from build123d import *
from build123d.topology import SkipClean

# Parameters (mm, degrees)
BOSS_EXTRUDE1_DEPTH = 5
BOSS_EXTRUDE2_DEPTH = 5
SKETCH4_R           = 1.5
SKETCH4_W           = 21.014084041
SKETCH4_H           = 55
SKETCH4_W_2         = 12
SKETCH4_H_2         = 5
CUT_EXTRUDE1_DEPTH  = 5
CIRPATTERN1_COUNT   = 3
SKETCH5_R           = 188.544827525
CUT_EXTRUDE2_DEPTH  = 5
BOSS_EXTRUDE3_START = -5
BOSS_EXTRUDE3_DEPTH = 5
BOSS_EXTRUDE4_START = -5
BOSS_EXTRUDE4_DEPTH = 5
BOSS_EXTRUDE5_START = -5
BOSS_EXTRUDE5_DEPTH = 5
CUT_EXTRUDE3_DEPTH  = 5
SKETCH8_R           = 1.5
SKETCH8_W           = 5
SKETCH8_H           = 15
CUT_EXTRUDE4_DEPTH  = 10
CIRPATTERN2_COUNT   = 3


with BuildPart() as part:
    # Sketch1 → Boss-Extrude1 (new body)
    with BuildSketch(Plane.XY):
        with BuildLine():
            Line((-8.818414939, -40.273942716), (-43.818414939, -100.895720981))
            ThreePointArc((-43.818414939, -100.895720981), (55, -95.262794416), (109.287464972, -12.5))
            Line((109.287464972, -12.5), (39.287464972, -12.5))
            Line((39.287464972, -12.5), (39.287464972, 12.5))
            Line((39.287464972, 12.5), (109.287464972, 12.5))
            ThreePointArc((109.287464972, 12.5), (55, 95.262794416), (-43.818414939, 100.895720981))
            Line((-43.818414939, 100.895720981), (-8.818414939, 40.273942716))
            Line((-8.818414939, 40.273942716), (-30.469050033, 27.773942716))
            Line((-30.469050033, 27.773942716), (-65.469050033, 88.395720981))
            ThreePointArc((-65.469050033, 88.395720981), (-110, 0), (-65.469050033, -88.395720981))
            Line((-65.469050033, -88.395720981), (-30.469050033, -27.773942716))
            Line((-30.469050033, -27.773942716), (-8.818414939, -40.273942716))
        make_face()
    extrude(amount=BOSS_EXTRUDE1_DEPTH)

    # Sketch3 → Boss-Extrude2 (add)
    with BuildSketch(Plane.XY.offset(5)):
        with BuildLine():
            Line((145.507042021, -22.5), (145.507042021, 22.5))
            ThreePointArc((145.507042021, 22.5), (141.113643739, 33.106601718), (130.507042021, 37.5))
            Line((130.507042021, 37.5), (96.507042021, 37.5))
            Line((96.507042021, 37.5), (96.507042021, -37.5))
            Line((96.507042021, -37.5), (130.507042021, -37.5))
            ThreePointArc((130.507042021, -37.5), (141.113643739, -33.106601718), (145.507042021, -22.5))
        make_face()
        with BuildLine():
            Line((120.507042021, -27.5), (106.507042021, -27.5))
            Line((106.507042021, -27.5), (106.507042021, 27.5))
            Line((106.507042021, 27.5), (120.507042021, 27.5))
            ThreePointArc((120.507042021, 27.5), (131.113643739, 23.106601718), (135.507042021, 12.5))
            Line((135.507042021, 12.5), (135.507042021, -12.5))
            ThreePointArc((135.507042021, -12.5), (131.113643739, -23.106601718), (120.507042021, -27.5))
        make_face(mode=Mode.SUBTRACT)
    boss_extrude2 = extrude(amount=-BOSS_EXTRUDE2_DEPTH)

    # Sketch4 → Cut-Extrude1 (cut)
    with BuildSketch(Plane.XY.offset(5)):
        with Locations((72.5, -20.5)):
            Circle(SKETCH4_R)
        with Locations((72.5, 20.5)):
            Circle(SKETCH4_R)
        with Locations((47.5, 20.5)):
            Circle(SKETCH4_R)
        with Locations((47.5, -20.861898396)):
            Circle(SKETCH4_R)
        with Locations((106.50704202, 0)):
            Rectangle(SKETCH4_W, SKETCH4_H)
        with Locations((85, -20.5)):
            Rectangle(SKETCH4_W_2, SKETCH4_H_2)
        with Locations((60, -20.5)):
            Rectangle(SKETCH4_W_2, SKETCH4_H_2)
        with Locations((85, 20.5)):
            Rectangle(SKETCH4_W_2, SKETCH4_H_2)
        with Locations((60, 20.5)):
            Rectangle(SKETCH4_W_2, SKETCH4_H_2)
    cut_extrude1 = extrude(amount=-CUT_EXTRUDE1_DEPTH, mode=Mode.SUBTRACT)

    # CirPattern1: Boss-Extrude2, Cut-Extrude1 ×3 about axis
    cirpattern1_axis = Axis((0, 0, 0), (0, 0, 1))
    add([boss_extrude2.rotate(cirpattern1_axis, i * 360 / CIRPATTERN1_COUNT) for i in range(1, CIRPATTERN1_COUNT)])
    add([cut_extrude1.rotate(cirpattern1_axis, i * 360 / CIRPATTERN1_COUNT) for i in range(1, CIRPATTERN1_COUNT)], mode=Mode.SUBTRACT)

    # Sketch5 → Cut-Extrude2 (cut)
    with BuildSketch(Plane.XY.offset(5)):
        with Locations((130.507042021, 226.044827525)):
            Circle(SKETCH5_R)
    extrude(amount=-CUT_EXTRUDE2_DEPTH, mode=Mode.SUBTRACT)

    # Sketch5_2 → Boss-Extrude3 (add)
    with SkipClean():  # the faces are left unmerged after this step: merging them gives an invalid solid
        with BuildSketch(Plane.XY.offset(5).offset(BOSS_EXTRUDE3_START)):
            with BuildLine():
                ThreePointArc((-17.04807225, 108.670894137), (-25.34145383, 119.929803482), (-32.777568368, 131.772413763))
                Line((-32.777568368, 131.772413763), (-19.229342058, 108.30619744))
                ThreePointArc((-19.229342058, 108.30619744), (-18.139623705, 108.494027724), (-17.04807225, 108.670894137))
            make_face()
            with BuildLine():
                Line((103.4105894, 37.5), (130.507042021, 37.5))
                ThreePointArc((130.507042021, 37.5), (116.532983402, 38.018558956), (102.6357911, 39.571383414))
                ThreePointArc((102.6357911, 39.571383414), (103.02839602, 38.537638919), (103.4105894, 37.5))
            make_face()
        extrude(amount=BOSS_EXTRUDE3_DEPTH)

    # Sketch6 → Boss-Extrude4 (add)
    with SkipClean():  # the faces are left unmerged after this step: merging them gives an invalid solid
        with BuildSketch(Plane.XY.offset(5).offset(BOSS_EXTRUDE4_START)):
            with BuildLine():
                add(Edge.make_bspline(
                    [(139.712182128, -34.343369267), (99.956513164, -69.307138706), (55.000005485, -95.262791249)],
                    knots=[0.008670154, 0.008670154, 0.008670154, 0.49999997, 0.49999997, 0.49999997], degree=2))
                ThreePointArc((139.712182128, -34.343369267), (135.372710576, -36.688913613), (130.507042021, -37.5))
                Line((130.507042021, -37.5), (103.4105894, -37.5))
                ThreePointArc((103.4105894, -37.5), (84.306667329, -70.656817391), (55.000005485, -95.262791249))
            make_face()
            with BuildLine():
                ThreePointArc((-32.777568368, -131.772413763), (-35.912824062, -135.580663145), (-40.113860827, -138.165983575))
                add(Edge.make_bspline(
                    [(55.000005485, -95.262791249), (10.043492321, -121.218446959), (-40.113860827, -138.165983575)],
                    knots=[0.49999997, 0.49999997, 0.49999997, 0.991329846, 0.991329846, 0.991329846], degree=2))
                ThreePointArc((55.000005485, -95.262791249), (19.037271385, -108.340123215), (-19.229342058, -108.30619744))
                Line((-19.229342058, -108.30619744), (-32.777568368, -131.772413763))
            make_face()
            with BuildLine():
                add(Edge.make_bspline(
                    [(-110, -5.52e-07), (-109.999999945, -51.91130743), (-99.598321301, -103.822614307)],
                    knots=[0.500000003, 0.500000003, 0.500000003, 0.991329846, 0.991329846, 0.991329846], degree=2))
                ThreePointArc((-99.598321301, -103.822614307), (-99.459886514, -98.891749532), (-97.729473652, -94.272413763))
                Line((-97.729473652, -94.272413763), (-84.181247342, -70.80619744))
                ThreePointArc((-84.181247342, -70.80619744), (-103.343933466, -37.683304204), (-110, -5.52e-07))
            make_face()
            with BuildLine():
                ThreePointArc((-97.729473652, 94.272413763), (-99.459886514, 98.891749532), (-99.598321301, 103.822614307))
                add(Edge.make_bspline(
                    [(-99.598321301, 103.822614307), (-110.000000055, 51.911306877), (-110, -5.52e-07)],
                    knots=[0.008670154, 0.008670154, 0.008670154, 0.500000003, 0.500000003, 0.500000003], degree=2))
                ThreePointArc((-110, -5.52e-07), (-103.343933655, 37.683303685), (-84.181247342, 70.80619744))
                Line((-84.181247342, 70.80619744), (-97.729473652, 94.272413763))
            make_face()
        extrude(amount=BOSS_EXTRUDE4_DEPTH)

    # Sketch7 → Boss-Extrude5 (add)
    with BuildSketch(Plane(origin=(0, 0, 0), x_dir=(-1, 0, 0), z_dir=(0, 0, -1)).offset(BOSS_EXTRUDE5_START)):
        with BuildLine():
            Line((-155.507042021, 22.5), (-155.507042021, -22.5))
            ThreePointArc((-155.507042021, -22.5), (-153.037379973, -33.334383774), (-146.11633228, -42.028186234))
            add(Edge.make_bspline(
                [(36.660689186, -147.554548779), (2.706672334, -136.063921523), (-29.525971209, -121.51723718), (-90.474028791, -86.328859728), (-119.188148744, -65.68791376), (-146.11633228, -42.028186234)],
                knots=[0, 0, 0, 0, 0.5, 0.5, 1, 1, 1, 1], degree=3))
            ThreePointArc((36.660689186, -147.554548779), (47.650266819, -149.201450672), (58.267949425, -145.923048857))
            Line((58.267949425, -145.923048857), (97.239092596, -123.423048857))
            ThreePointArc((97.239092596, -123.423048857), (105.387113154, -115.867066899), (109.455643094, -105.526362546))
            add(Edge.make_bspline(
                [(109.455643094, 105.526362546), (116.48147641, 70.376007763), (120, 35.188377452), (120, -35.188377452), (116.48147641, -70.376007763), (109.455643094, -105.526362546)],
                knots=[0, 0, 0, 0, 0.5, 0.5, 1, 1, 1, 1], degree=3))
            ThreePointArc((109.455643094, 105.526362546), (105.387113154, 115.867066899), (97.239092596, 123.423048857))
            Line((97.239092596, 123.423048857), (58.267949425, 145.923048857))
            ThreePointArc((58.267949425, 145.923048857), (46.474352087, 145.735057462), (38.267949425, 137.262794819))
            ThreePointArc((38.267949425, 137.262794819), (45.767949425, 139.272413763), (53.267949425, 137.262794819))
            Line((53.267949425, 137.262794819), (92.239092596, 114.762794819))
            ThreePointArc((92.239092596, 114.762794819), (97.185203012, 110.144649755), (99.598321301, 103.822614307))
            add(Edge.make_bspline(
                [(99.598321301, -103.822614309), (120.401678699, -1e-09), (99.598321301, 103.822614307)],
                knots=[0, 0, 0, 1, 1, 1], degree=2))
            ThreePointArc((99.598321301, -103.822614309), (97.185203011, -110.144649756), (92.239092596, -114.762794819))
            Line((92.239092596, -114.762794819), (53.267949425, -137.262794819))
            ThreePointArc((53.267949425, -137.262794819), (46.795463273, -139.237179557), (40.113860827, -138.165983575))
            add(Edge.make_bspline(
                [(-139.712182129, -34.343369266), (-60.20083935, -104.270912411), (40.113860827, -138.165983575)],
                knots=[0, 0, 0, 1, 1, 1], degree=2))
            ThreePointArc((-139.712182129, -34.343369266), (-143.980666285, -29.092529802), (-145.507042021, -22.5))
            Line((-145.507042021, -22.5), (-145.507042021, 22.5))
            ThreePointArc((-145.507042021, 22.5), (-143.497423077, 30), (-138.007042021, 35.490381057))
            ThreePointArc((-138.007042021, 35.490381057), (-149.447438028, 32.619559199), (-155.507042021, 22.5))
        make_face()
        with BuildLine():
            ThreePointArc((29.086468731, 125.650289264), (-39.369546298, 68.190054459), (-123.359576861, 37.635523805))
            ThreePointArc((-123.359576861, 37.635523805), (-36.234628258, 62.760217136), (29.086468731, 125.650289264))
        make_face()
    extrude(amount=BOSS_EXTRUDE5_DEPTH)

    # Sketch7_3 → Cut-Extrude3 (cut)
    with BuildSketch(Plane(origin=(0, 0, 0), x_dir=(-1, 0, 0), z_dir=(0, 0, -1))):
        with BuildLine():
            ThreePointArc((32.777568368, 131.772413763), (30.961036496, 128.693856258), (29.086468731, 125.650289264))
            ThreePointArc((29.086468731, 125.650289264), (33.760803526, 131.390447709), (38.267949425, 137.262794819))
            ThreePointArc((38.267949425, 137.262794819), (35.161347707, 134.87901548), (32.777568368, 131.772413763))
        make_face()
        with BuildLine():
            ThreePointArc((-130.507042021, 37.5), (-134.389327697, 36.988887394), (-138.007042021, 35.490381057))
            ThreePointArc((-138.007042021, 35.490381057), (-130.667867293, 36.457510349), (-123.359576861, 37.635523805))
            ThreePointArc((-123.359576861, 37.635523805), (-126.932667079, 37.533883996), (-130.507042021, 37.5))
        make_face()
    extrude(amount=-CUT_EXTRUDE3_DEPTH, mode=Mode.SUBTRACT)

    # Sketch8 → Cut-Extrude4 (cut)
    with BuildSketch(Plane(origin=(0, 0, 0), x_dir=(-1, 0, 0), z_dir=(0, 0, -1))):
        with Locations((-140.507042021, 16)):
            Circle(SKETCH8_R)
        with Locations((-140.507042021, -16)):
            Circle(SKETCH8_R)
        with Locations((-150.507042021, -16)):
            Circle(SKETCH8_R)
        with Locations((-150.507042021, 16)):
            Circle(SKETCH8_R)
        with Locations((-145.507042021, 0)):
            Rectangle(SKETCH8_W, SKETCH8_H)
    cut_extrude4 = extrude(amount=-CUT_EXTRUDE4_DEPTH, mode=Mode.SUBTRACT)

    # CirPattern2: Cut-Extrude4 ×3 about axis
    cirpattern2_axis = Axis((0, 0, 0), (0, 0, 1))
    for i in range(1, CIRPATTERN2_COUNT):
        add(cut_extrude4.rotate(cirpattern2_axis, i * 360 / CIRPATTERN2_COUNT), mode=Mode.SUBTRACT)


solid = part.part
Source: CAD feature listing. Evaluate the final solid. Frame: model axes, mm. A direction names the side the tool comes from. Coordinates: 2 decimals unless noted, no trailing zeros. Write each question's results on one line, items separated by ' | '. Start each with the question number.
1. Section A-A, the plane z = 3.75. State how many separate pieces and enclosed holes the cut face has, then the cut area to 3 significant figures.
2. Reachability of faces 1 (the face through (-67.905, 117.265, 2.535)), 2 (the face through (-105.298, -115.996, 2.535)) from +Z, -Z, +X, -X, +Y, -Y: full face, straight path, thin tool, end or side. Return the list, or none.
3. Pin query (flat end, axial travel): pin 1 (1.5 mm diameter, centred on x = 86, z = 3.5, fed in from +Y). Return the tip coordinate at first contact, or that it passes through.
4. Material intervals for L1, parallel to X at y = 2, z = 1.1; L2, parallel to Y at x = 60, z = 4.65; L3, parallel to Y at x = 47.5, z = 3.95, sorted ascending.
Solution:
1) separate pieces: 1 | enclosed holes: 42 | area: 41,400 mm²
2) face 1: +Z, -Z | face 2: +Z, -Z, -X, -Y
3) pin 1: y = 47.4
4) L1: -120 to 39.29, 135.51 to 143.01, 148.01 to 155.51 | L2: -103.92 to -23, -18 to -12.5, 12.5 to 18, 23 to 57.49 | L3: -110.92 to -22.36, -19.36 to -12.5, 12.5 to 19, 22 to 63.69
